Source: CAD feature listing. Evaluate the final solid. Frame: model axes, mm. Face numbers are marked on the shaded views. A direction names the side the tool comes from. Coordinates: 2 decimals unless noted, no trailing zeros. Write each loop counter-clockwise with the first axis right and the second up, starting at its lowest first coordinate (ties: lowest second). Pieces come first, ordered by that corner, then holes. Notation, with made-up numbers: (29.5, 40.25) -> (64.5, 40.25) arc R10 cw to (64.5, 57.25) -> close; hole circle Ø5 at (84.5, 28.25). An arc over 180 degrees is marked (long way). One line per item, written item: value. Start each with the question number.
1. First-contact query: P1, Ø8, axis at x = -33.5, z = -1, coming from the +Y side; P2, Ø0.7, axis at y = 10, z = -11, coming from the -X side; P3, Ø8, axis at x = 40, z = -8.5, coming from the +Y side; P4, Ø3, axis at x = -8, y = 9, coming from the +Z side. Flat tips, straight axial feed; report the tip coordinate or a pass-through.
2. Mould query, pull axis X, two halves, no side actions, for the marked faces 1, 2, 3 and 4. Classes: released by +X, released by -X, zero draft, split by the parting line, or undercut.
3. Access query for the marked faces 5, 6 and 7. Directions: +Z, -Z, +X, -X, +Y, -Y. A direction counts if a zero-diameter tool reaches every point of the face in a straight line with its end or side. Return the directions, or none.
4. Section query D-D, the plane x = -15.5. Output: boundary loops of the cut face in (y, z), and give its area (3 significant figures).
5. Section query B-B, the plane x = 30.5. State how many separate pieces and enclosed holes the cut face has, and give its area (3 significant figures).
6. Line query: line 1 (Z direction, x = 44, y = 2.5) (3 decimals); line 2 (X direction, y = 2.25, z = 3.25); line 3 (X direction, y = 2, z = -8.25). Output: solid intervals per line, ascending.
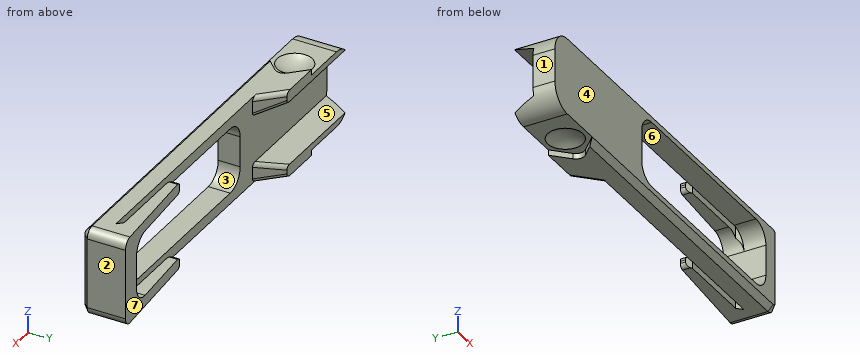
from build123d import *

# Parameters (mm, degrees)
BOSS_EXTRUDE1_DEPTH = 12.7
SKETCH2_W           = 19.05
SKETCH2_H           = 6.35
CUT_EXTRUDE1_DEPTH  = 107.95
CUT_EXTRUDE2_DEPTH  = 64.816710194
CHAMFER1_SIZE       = 6.978592645
CHAMFER1_SIZE_2     = 2.54
CUT_EXTRUDE3_DEPTH  = 1.5875
CHAMFER3_SIZE       = 1.5875
FILLET1_R           = 6.35
FILLET2_R           = 1.27
FILLET3_R           = 5.08
CHAMFER4_SIZE       = 1.524
CUT_EXTRUDE4_DEPTH  = 59.887477446


# Some blends are built 0.0001 mm under size
with BuildPart() as part:
    # Sketch1 → Boss-Extrude1 (new body)
    with BuildSketch(Plane(origin=(0, 0, 0), x_dir=(1, 0, 0), z_dir=(0, 1, 0))):
        with BuildLine():
            Line((-50.8, 12.7), (-57.15, 12.7))
            Line((-57.15, 12.7), (-57.15, 6.35))
            Line((-57.15, 6.35), (-57.15, -6.35))
            Line((-57.15, -6.35), (-57.15, -12.7))
            Line((-57.15, -12.7), (-50.8, -12.7))
            Line((-50.8, -12.7), (54.61, -12.7))
            ThreePointArc((54.61, -12.7), (56.406051224, -11.956051224), (57.15, -10.16))
            Line((57.15, -10.16), (57.15, 10.16))
            ThreePointArc((57.15, 10.16), (56.406051224, 11.956051224), (54.61, 12.7))
            Line((54.61, 12.7), (-50.8, 12.7))
        make_face()
    extrude(amount=BOSS_EXTRUDE1_DEPTH)

    # Sketch2 → Cut-Extrude1 (cut)
    with BuildSketch(Plane.ZY.offset(57.15)):
        with Locations((0, 9.525)):
            Rectangle(SKETCH2_W, SKETCH2_H)
    extrude(amount=-CUT_EXTRUDE1_DEPTH, mode=Mode.SUBTRACT)

    # Sketch3 → Cut-Extrude2 (cut, through all)
    with BuildSketch(Plane.XY.offset(12.7)):
        Polygon((25.4, 10.414), (57.15, 12.7), (-25.4, 12.7), (-19.05, 6.35), (50.8, 6.35), (50.8, 7.874), (27.15976362, 7.874), (25.4, 8.89), align=None)
    extrude(amount=-CUT_EXTRUDE2_DEPTH, mode=Mode.SUBTRACT)

    # Chamfer1
    # the kernel refuses this chamfer: 6.978592645, 2.54 mm, written as the material it adds along each edge
    with BuildSketch(Plane(origin=(-57.15, 6.35, 9.525), x_dir=(0, 0.9999130865277316, 0.013184058198642549), z_dir=(1, 0, 0))) as chamfer1_piece_1_section:
        Polygon((CHAMFER1_SIZE * 0.999913086587, -CHAMFER1_SIZE * 0.0131840581994), (-CHAMFER1_SIZE_2 * 0.0131840581987, -CHAMFER1_SIZE_2 * 0.999913086528), (0, 0), align=None)
    chamfer1_piece_1 = extrude(amount=56.203828281, mode=Mode.PRIVATE)
    chamfer1_piece_1 = split(chamfer1_piece_1, bisect_by=Plane(origin=(-39.199121236, 12.7, 8.706690515), z_dir=(0, -1, 0)), keep=Keep.TOP, mode=Mode.PRIVATE)
    chamfer1_piece_1 = split(chamfer1_piece_1, bisect_by=Plane(origin=(-30.223681853, 17.523681853, 8.706690515), z_dir=(-0.7071067811865448, -0.7071067811865503, 0)), keep=Keep.TOP, mode=Mode.PRIVATE)
    add(chamfer1_piece_1)
    with BuildSketch(Plane(origin=(-57.15, 6.35, -9.525), x_dir=(0, -0.09904090225207035, 0.9950833631817466), z_dir=(1, 0, 0))) as chamfer1_piece_2_section:
        Polygon((CHAMFER1_SIZE_2 * 0.995083363182, -CHAMFER1_SIZE_2 * 0.099040902252), (-CHAMFER1_SIZE * 0.099040902258, -CHAMFER1_SIZE * 0.995083363241), (0, 0), align=None)
    chamfer1_piece_2 = extrude(amount=56.203828281, mode=Mode.PRIVATE)
    chamfer1_piece_2 = split(chamfer1_piece_2, bisect_by=Plane(origin=(-30.223681853, 17.523681853, -8.706690515), z_dir=(-0.7071067811865448, -0.7071067811865503, 0)), keep=Keep.TOP, mode=Mode.PRIVATE)
    chamfer1_piece_2 = split(chamfer1_piece_2, bisect_by=Plane(origin=(-39.199121236, 12.7, -8.706690515), z_dir=(0, -1, 0)), keep=Keep.TOP, mode=Mode.PRIVATE)
    add(chamfer1_piece_2)

    # Sketch4 → Cut-Extrude3 (cut)
    with BuildSketch(Plane.XY.offset(12.7)):
        with BuildLine():
            Line((-57.15, 12.7), (-57.15, 0))
            Line((-57.15, 0), (-38.1, 0))
            Line((-38.1, 0), (-33.546051224, 4.553948776))
            ThreePointArc((-33.546051224, 4.553948776), (-32.802102448, 6.35), (-33.546051224, 8.146051224))
            Line((-33.546051224, 8.146051224), (-38.1, 12.7))
            Line((-38.1, 12.7), (-57.15, 12.7))
        make_face()
    cut_extrude3 = extrude(amount=-CUT_EXTRUDE3_DEPTH, mode=Mode.SUBTRACT)

    # Sketch6 → Cut-Revolve1 (revolve, cut)
    with BuildSketch(Plane.ZY.offset(40.64)):
        with BuildLine():
            Line((11.1125, 6.35), (11.1125, 11.43))
            ThreePointArc((11.1125, 11.43), (9.931118256, 9.01113492), (9.525, 6.35))
            Line((9.525, 6.35), (11.1125, 6.35))
        make_face()
    cut_revolve1 = revolve(axis=Axis((-40.64, 6.35, 12.7), (0, 0, -1)), mode=Mode.SUBTRACT)

    # Mirror1: Cut-Extrude3, Cut-Revolve1 across plane
    add(cut_extrude3.mirror(Plane(origin=(0, 0, 0), x_dir=(1, 0, 0), z_dir=(0, 0, -1))), mode=Mode.SUBTRACT)
    add(cut_revolve1.mirror(Plane(origin=(0, 0, 0), x_dir=(1, 0, 0), z_dir=(0, 0, -1))), mode=Mode.SUBTRACT)

    # Chamfer3
    chamfer3_edges = [part.edges().sort_by_distance(p)[0] for p in [
        (8.255, 0, 12.7),
        (56.406051224, 0, 11.956051224),
        (57.15, 0, 0),
        (56.406051224, 0, -11.956051224),
        (8.255, 0, -12.7),
    ]]
    chamfer(chamfer3_edges, length=CHAMFER3_SIZE)

    # Fillet1
    fillet1_edges = [part.edges().sort_by_distance(p)[0] for p in [
        (-57.15, 6.35, -11.1125),
        (-57.15, 6.35, 11.1125),
    ]]
    fillet(fillet1_edges, radius=FILLET1_R)

    # Fillet2
    fillet2_edges = [part.edges().sort_by_distance(p)[0] for p in [
        (-22.225, 9.525, 8.140605494),
        (-22.225, 9.525, -8.140605494),
        (25.4, 9.652, -9.525),
        (-22.225, 9.525, 12.7),
        (25.4, 9.652, 12.7),
        (25.4, 9.652, 9.525),
        (25.4, 9.652, -12.7),
        (-22.225, 9.525, -12.7),
    ]]
    fillet(fillet2_edges, radius=FILLET2_R)

    # Fillet3
    fillet3_edges = [part.edges().sort_by_distance(p)[0] for p in [
        (50.8, 10.0584, -9.525),
        (50.8, 10.0584, 9.525),
    ]]
    fillet(fillet3_edges, radius=FILLET3_R)

    # Chamfer4
    chamfer4_edges = [part.edges().sort_by_distance(p)[0] for p in [
        (50.8, 7.874, -8.5725),
        (50.8, 7.874, 8.5725),
    ]]
    chamfer(chamfer4_edges, length=CHAMFER4_SIZE - 0.0001)  # a hair under: the kernel refuses the full size

    # Sketch7 → Cut-Extrude4 (cut, through all)
    with BuildSketch(Plane(origin=(0, 6.35, 0), x_dir=(1, 0, 0), z_dir=(0, 1, 0))):
        with BuildLine():
            Line((26.67, -9.525), (45.72, -9.525))
            ThreePointArc((45.72, -9.525), (49.312102448, -8.037102448), (50.8, -4.445))
            Line((50.8, -4.445), (50.8, 4.445))
            ThreePointArc((50.8, 4.445), (49.312102448, 8.037102448), (45.72, 9.525))
            Line((45.72, 9.525), (26.67, 9.525))
            Line((26.67, 9.525), (-7.62, 9.525))
            ThreePointArc((-7.62, 9.525), (-11.212102448, 8.037102448), (-12.7, 4.445))
            Line((-12.7, 4.445), (-12.7, -4.445))
            ThreePointArc((-12.7, -4.445), (-11.212102448, -8.037102448), (-7.62, -9.525))
            Line((-7.62, -9.525), (26.67, -9.525))
        make_face()
    extrude(amount=-CUT_EXTRUDE4_DEPTH, mode=Mode.SUBTRACT)


solid = part.part
Computed values:
1. P1: stops at y = 6.35
1. P2: stops at x = -53.18
1. P3: stops at y = 11.74
1. P4: passes through
2. face 1: released by -X
2. face 2: released by +X
2. face 3: undercut
2. face 4: zero draft
3. face 5: -X, +Y
3. face 6: +Y, -Y
3. face 7: +Z, -Z, +Y
4. outline: (0, -11.11) -> (1.59, -12.7) -> (6.35, -12.7) -> (6.35, 12.7) -> (1.59, 12.7) -> (0, 11.11) -> close
4. area: 159 mm²
5. separate pieces: 4
5. enclosed holes: 0
5. area: 56.3 mm²
6. line 1: z = -12.7 to -9.525, 9.525 to 12.7
6. line 2: x = -57.15 to -12.7, 50.8 to 57.15
6. line 3: x = -56.11 to -10.99, 49.09 to 57.15
